```python
from build123d import *

# Parameters (mm, degrees)
BOSS_EXTRUDE1_DEPTH = 22.5
SKETCH2_R           = 20
SKETCH2_R_2         = 37.5
CUT_EXTRUDE2_DEPTH  = 11
FILLET1_R           = 8
SKETCH3_R           = 6
SKETCH3_R_2         = 4
CUT_EXTRUDE3_DEPTH  = 44.5
CUT_EXTRUDE6_DEPTH  = 1.5
BOSS_EXTRUDE2_DEPTH = 1.5


with BuildPart() as part:
    # Sketch1 → Boss-Extrude1 (new, symmetric)
    with BuildSketch(Plane(origin=(0, 0, 0), x_dir=(1, 0, 0), z_dir=(0, 1, 0))):
        with BuildLine():
            Line((-90.833333333, 14.976833963), (-1.111111111, 19.969111951))
            ThreePointArc((-1.111111111, 19.969111951), (20, 0), (-1.111111111, -19.969111951))
            Line((-1.111111111, -19.969111951), (-90.833333333, -14.976833963))
            ThreePointArc((-90.833333333, -14.976833963), (-105, 0), (-90.833333333, 14.976833963))
        make_face()
    extrude(amount=BOSS_EXTRUDE1_DEPTH, both=True)

    # Sketch2 → Cut-Extrude2 (cut)
    with BuildSketch(Plane(origin=(0, 22.5, 0), x_dir=(1, 0, 0), z_dir=(0, 1, 0))):
        with Locations((-90, 0)):
            Circle(SKETCH2_R)
        Circle(SKETCH2_R_2)
    cut_extrude2 = extrude(amount=-CUT_EXTRUDE2_DEPTH, mode=Mode.SUBTRACT)

    # Mirror1: Cut-Extrude2 across plane
    add(cut_extrude2.mirror(Plane.ZX), mode=Mode.SUBTRACT)

    # Fillet1
    fillet1_edges = [part.edges().sort_by_distance(p)[0] for p in [
        (-55.204285794, 22.5, 16.959287199),
        (-55.204285794, 22.5, -16.959287199),
        (-55.204285794, -22.5, 16.959287199),
        (-55.204285794, -22.5, -16.959287199),
    ]]
    fillet(fillet1_edges, radius=FILLET1_R)

    # Sketch3 → Cut-Extrude3 (cut)
    with BuildSketch(Plane(origin=(0, 11.5, 0), x_dir=(1, 0, 0), z_dir=(0, 1, 0))):
        with Locations(Location((0, 0, 0), (0, 0, 270))):
            Circle(SKETCH3_R)
        with Locations(Location((-90, 0, 0), (0, 0, 270))):
            Circle(SKETCH3_R_2)
    extrude(amount=-CUT_EXTRUDE3_DEPTH, mode=Mode.SUBTRACT)

    # Sketch5 → Cut-Extrude6 (cut)
    with BuildSketch(Plane(origin=(0, 22.5, 0), x_dir=(1, 0, 0), z_dir=(0, 1, 0))):
        Polygon((-55, -7.505553499), (-48.5, -3.75277675), (-48.5, 3.75277675), (-55, 7.505553499), (-61.5, 3.75277675), (-61.5, -3.75277675), align=None)
    cut_extrude6 = extrude(amount=-CUT_EXTRUDE6_DEPTH, mode=Mode.SUBTRACT)

    # Sketch6 → Boss-Extrude2 (add)
    with BuildSketch(Plane(origin=(0, 22.5, 0), x_dir=(1, 0, 0), z_dir=(0, 1, 0))):
        with BuildLine():
            Line((-64.640723816, 2.716865752), (-64.640723816, -2.567368827))
            ThreePointArc((-64.640723816, -2.567368827), (-66.140723816, -4.067368827), (-67.640723816, -2.567368827))
            Line((-67.640723816, -2.567368827), (-67.640723816, 2.716865752))
            ThreePointArc((-67.640723816, 2.716865752), (-66.140723816, 4.216865752), (-64.640723816, 2.716865752))
        make_face()
        with BuildLine():
            Line((-41.5, 2.726821799), (-41.5, -2.55741278))
            ThreePointArc((-41.5, -2.55741278), (-43, -4.05741278), (-44.5, -2.55741278))
            Line((-44.5, -2.55741278), (-44.5, 2.726821799))
            ThreePointArc((-44.5, 2.726821799), (-43, 4.226821799), (-41.5, 2.726821799))
        make_face()
    boss_extrude2 = extrude(amount=BOSS_EXTRUDE2_DEPTH)

    # Mirror2: Cut-Extrude6, Boss-Extrude2 across plane
    add(cut_extrude6.mirror(Plane.ZX), mode=Mode.SUBTRACT)
    add(boss_extrude2.mirror(Plane.ZX))


solid = part.part
```
CAD build for the part. Positions are in the model's coordinates, mm. A direction names the side the tool comes from. Coordinates: 2 decimals unless noted, no trailing zeros. Loops run counter-clockwise (first coordinate to the right, second up) from the corner with the lowest first, then second, coordinate; pieces in that order, holes last. Notation, with made-up numbers: (77.25, 11) - (128.25, 11) arc R35 ccw to (128.25, 49) - close; hole circle Ø7 at (48.5, 59). An arc over 180 degrees is marked (long way). Return JSON: item names as keys, results as strings.
1. Probe L1, parallel to X at y = -2.75, z = 0; L2, parallel to Y at x = -66, z = -8; L3, parallel to Y at x = -8.5, z = 9.5. List the from-to ranges inside material, lowest first. Write a range as from..to.
Result:
{"L1": "x = -105..-94, -86..-6, 6..20", "L2": "y = -22.5..22.5", "L3": "y = -11.5..11.5"}
2. 3-axis set-ups, long thin cutter, end or side, ignore diameter. For faces 1 (the flat face through (-84, 11.5, 0)), 2 (the flat face through (-58.2, -21.76, -5.66)), 3 (the flat face through (-51.8, 21.76, 5.66)), 4 (the cylindrical face through (-37.5, 17.1, -0.3)): which of +Z, -Z, +X, -X, +Y, -Y reach the whole face in a straight line?
Result:
{"face 1": "-X, +Y", "face 2": "-Y", "face 3": "+Y", "face 4": "+X, +Y"}
3. Mould opens along X. For faces 5 (the flat face through (-9, -11.5, 0)), 6 (the flat face through (-58.3, 21.8, 5.6)), 7 (the flat face through (-55, -21, 0)), 8 (the flat face through (-46.6, 0.2, -17.44)) say: released by +X, released by -X, zero draft, split by the parting line, or undercut.
Result:
{"face 5": "zero draft", "face 6": "undercut", "face 7": "undercut", "face 8": "released by -X"}
4. Band-saw the part on C-C (x = -15). Give the cut face in (y, z), and give its area (3 significant figures).
Result:
{"outline": "(-11.5, -19.2) - (11.5, -19.2) - (11.5, 19.2) - (-11.5, 19.2) - close", "area": "883 mm2"}
5. Band-saw the part on B-B (z = 0). State how many separate pieces and enclosed holes the cut face has, and give its area (3 significant figures).
Result:
{"separate pieces": "3", "enclosed holes": "0", "area": "3,110 mm2"}
6. Drop flat-ended pins along their axis: pin 1 (5 mm diameter, centred on x = -82, y = 12, fed in from +Z); pin 2 (5 mm diameter, centred on x = -84.5, y = 14.5, fed in from +Z); pin 3 (4 mm diameter, centred on x = -51, z = 10, fed in from +Y); pin 4 (13 mm diameter, centred on x = -90, z = 0, fed in from +Y). Give the stop position or say it passes through.
Result:
{"pin 1": "stops at z = 15.6", "pin 2": "passes through", "pin 3": "stops at y = 22.5", "pin 4": "stops at y = 11.5"}
7. Band-saw the part on A-A (y = 4). Give the cut face in (x, z), and give its area (3 significant figures).
Result:
{"outline": "(-90.83, -14.98) - (-1.11, -19.97) arc R20 ccw (long way) to (-1.11, 19.97) - (-90.83, 14.98) arc R15 ccw to start; hole circle Ø8 at (-90, 0); hole circle Ø12 at (0, 0)", "area": "3,970 mm2"}
8. Band-saw the part on D-D (y = -18). Give the cut face in (x, z).
Result:
{"outline": "(-76.72, -14.95) - (-33.23, -17.37) arc R37.5 cw to (-33.23, 17.37) - (-76.72, 14.95) arc R20 cw to start"}
